Input: part model. Units: mm. Frame: model coordinates. Face numbers are marked on the shaded views. A direction names the side the tool comes from. Coordinates: 2 decimals unless noted, no trailing zeros. Order: outer loops, then holes, each group sorted by start corner. A loop starts at its lowest first (then second) coordinate and runs counter-clockwise, first axis right, second up.
from build123d import *

# Parameters (mm, degrees)
F0_W     = 1524
F0_H     = 304.8
F1_DEPTH = 355.6
F2_T     = -3.175
F3_R     = 6.35
F4_DEPTH = 25.4


with BuildPart() as f1:
    # F0 (on Front) → F1 (new body)
    with BuildSketch(Plane.XZ):
        Rectangle(F0_W, F0_H)
    extrude(amount=F1_DEPTH)

    # F2
    f2_openings = [f1.faces().sort_by_distance(p)[0] for p in [
        (0, -177.8, 152.4),
    ]]
    offset(amount=F2_T, openings=f2_openings)

    # F3 (on face) → F4 (cut)
    with BuildSketch(Plane(origin=(0, 0, -152.4), x_dir=(1, 0, 0), z_dir=(0, 0, -1))):
        with Locations((-613.817692, 189.950407)):
            Circle(F3_R)
        with Locations((-461.417692, 189.950407)):
            Circle(F3_R)
        with Locations((-309.017692, 189.950407)):
            Circle(F3_R)
        with Locations((-156.617692, 189.950407)):
            Circle(F3_R)
        with Locations((-4.217692, 189.950407)):
            Circle(F3_R)
        with Locations((148.182308, 189.950407)):
            Circle(F3_R)
        with Locations((300.582308, 189.950407)):
            Circle(F3_R)
        with Locations((452.982308, 189.950407)):
            Circle(F3_R)
        with Locations((605.382308, 189.950407)):
            Circle(F3_R)
    extrude(amount=-F4_DEPTH, mode=Mode.SUBTRACT)


solid = f1.part
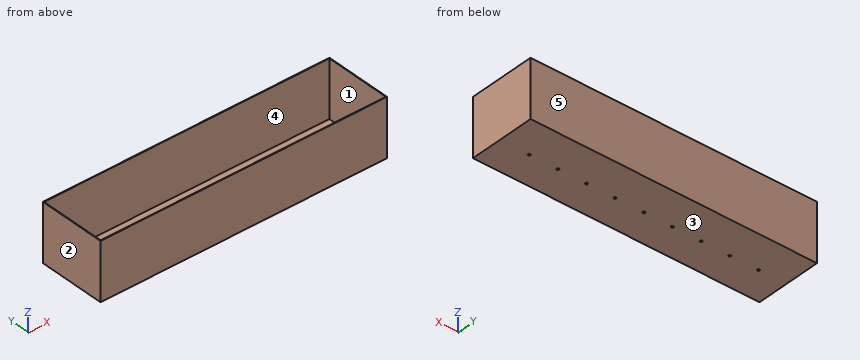
Item 1: Cut plane B-B on y = -224.5. Return loops of the section in (x, z) (3 decimals), then the cut area to 3 significant figures.
Response values:
outline: (-762, -152.4) - (762, -152.4) - (762, 152.4) - (758.825, 152.4) - (758.825, -149.225) - (-758.825, -149.225) - (-758.825, 152.4) - (-762, 152.4) - close
area: 6,750 mm2
Item 2: Pin query (flat end, axial travel): pin 1 Ø20.5 at (x, y) = (-461.42, -189.95) entering from +Z (3 decimals); pin 2 Ø11.5 at (x, y) = (-309.02, -189.95) entering from -Z. Return the tip coordinate at first contact, or that it passes through.
Response values:
pin 1: stops at z = -149.225
pin 2: passes through
Item 3: Ray query, probe 1 along X at (y, z) = (-138, 82.5) (3 decimals); probe 2 along Y at (x, z) = (366, -52.5) (3 decimals); probe 3 along Z at (x, y) = (-30.5, -193.5) (3 decimals). Return the intervals inside material, ascending.
Response values:
probe 1: x = -762 to -758.825, 758.825 to 762
probe 2: y = -355.6 to -352.425, -3.175 to 0
probe 3: z = -152.4 to -149.225
Item 4: Draft query along X for the marked faces 1, 2 and 3. Return one class per face: pulls with the +X half, pulls with the -X half, needs draft (parallel to the pull), parting line crosses it, or undercut.
Response values:
face 1: undercut
face 2: pulls with the -X half
face 3: needs draft
Item 5: Cut plane C-C on x = 191. Return loops of the section in (y, z) (3 decimals), then the cut area to 3 significant figures.
Response values:
outline: (-355.6, -152.4) - (0, -152.4) - (0, 152.4) - (-3.175, 152.4) - (-3.175, -149.225) - (-352.425, -149.225) - (-352.425, 152.4) - (-355.6, 152.4) - close
area: 3,040 mm2
Item 6: Cut plane A-A on z = -25. Return loops of the section in (x, y) (3 decimals).
Response values:
outline: (-762, -355.6) - (762, -355.6) - (762, 0) - (-762, 0) - close; hole (-758.825, -352.425) - (758.825, -352.425) - (758.825, -3.175) - (-758.825, -3.175) - close
Item 7: Access query for the marked faces 4 and 5. Directions: +Z, -Z, +X, -X, +Y, -Y. A direction counts if a zero-diameter tool reaches every point of the face in a straight line with its end or side. Return the directions, or none.
Response values:
face 4: +Z
face 5: +Z, -Z, +X, -X, +Y
